Work out the finished part from the listing and answer in its coordinate system (mm). A direction names the side the tool comes from. Round coordinates to 2 decimals unless told otherwise and drop trailing zeros. Loops run counter-clockwise (first coordinate to the right, second up) from the corner with the lowest first, then second, coordinate; pieces in that order, holes last. Notation, with made-up numbers: M 9,5.25 L 44,5.25 A18 ccw 44,33.25 Z; hole C 50.25,83 d5. An arc over 180 degrees is marked long. One line per item, written item: value.
```python
from build123d import *
from build123d.topology import SkipClean

# Parameters (mm, degrees)
BOSS_EXTRUDE4_DEPTH     = 6.35
BOSS_EXTRUDE5_START     = -34.925
BOSS_EXTRUDE5_OUTLINE_R = 19.05
BOSS_EXTRUDE5_DEPTH     = 34.925
SKETCH5_R               = 6.35
CUT_EXTRUDE1_DEPTH      = 12.7
SKETCH6_R               = 6.731
CUT_EXTRUDE2_DEPTH      = 12.7
SKETCH8_W               = 34.925
SKETCH8_H               = 7.9375
BOSS_EXTRUDE6_DEPTH     = 4.7625
SKETCH9_W               = 34.925
SKETCH9_H               = 7.9375
BOSS_EXTRUDE7_DEPTH     = 4.7625
FILLET1_R               = 12.7
FILLET1_OF_MIRROR1_R    = 12.7
SKETCH10_R              = 31.75
SKETCH10_R_2            = 19.05
BOSS_EXTRUDE8_DEPTH     = 44.45
BOSS_EXTRUDE9_DEPTH     = 12.7


# Read off the part's stored shape, not the designer's step: Boss-Extrude5
with BuildPart() as part:
    # Sketch2 → Boss-Extrude4 (new body)
    with BuildSketch(Plane.XY):
        with BuildLine():
            ThreePointArc((-12.522963776, 74.083126299), (-37.56705413, 31.749689456), (0, 0))
            Line((0, 0), (0, 6.35))
            ThreePointArc((0, 6.35), (-31.75, 38.1), (0, 69.85))
            Line((0, 69.85), (0, 76.2))
            ThreePointArc((0, 76.2), (-6.350310544, 75.66705413), (-12.522963776, 74.083126299))
        make_face()
        with BuildLine():
            Line((0, 6.35), (0, 0))
            ThreePointArc((0, 0), (26.940768363, 11.159231637), (38.1, 38.1))
            ThreePointArc((38.1, 38.1), (31.054266373, 60.173571076), (12.522963776, 74.083126299))
            ThreePointArc((12.522963776, 74.083126299), (6.350310544, 75.66705413), (0, 76.2))
            Line((0, 76.2), (0, 69.85))
            ThreePointArc((0, 69.85), (22.450640303, 60.550640303), (31.75, 38.1))
            ThreePointArc((31.75, 38.1), (22.450640303, 15.649359697), (0, 6.35))
        make_face()
        with BuildLine():
            ThreePointArc((38.1, 38.1), (26.940768363, 11.159231637), (0, 0))
            Line((0, 0), (88.9, 0))
            Line((88.9, 0), (88.9, 50.8))
            Line((88.9, 50.8), (12.522963776, 74.083126299))
            ThreePointArc((12.522963776, 74.083126299), (31.054266373, 60.173571076), (38.1, 38.1))
        make_face()
        with BuildLine():
            Line((-88.9, 0), (0, 0))
            ThreePointArc((0, 0), (-37.56705413, 31.749689456), (-12.522963776, 74.083126299))
            Line((-12.522963776, 74.083126299), (-88.9, 50.8))
            Line((-88.9, 50.8), (-88.9, 0))
        make_face()
    boss_extrude4 = extrude(amount=BOSS_EXTRUDE4_DEPTH)

    # Boss-Extrude5 outline → Boss-Extrude5 (add)
    with BuildSketch(Plane(origin=(0, 0, 0), x_dir=(-1, 0, 0), z_dir=(0, 0, -1)).offset(BOSS_EXTRUDE5_START)):
        with BuildLine():
            Line((101.6, 0), (101.6, 50.8))
            Line((101.6, 50.8), (88.9, 50.8))
            Line((88.9, 50.8), (88.9, 12.7))
            Line((88.9, 12.7), (31.75, 12.7))
            Line((31.75, 12.7), (31.75, 38.1))
            ThreePointArc((31.75, 38.1), (0, 69.85), (-31.75, 38.1))
            Line((-31.75, 38.1), (-31.75, 12.7))
            Line((-31.75, 12.7), (-88.9, 12.7))
            Line((-88.9, 12.7), (-88.9, 50.8))
            Line((-88.9, 50.8), (-101.6, 50.8))
            Line((-101.6, 50.8), (-101.6, 0))
            Line((-101.6, 0), (101.6, 0))
        make_face()
        with Locations((0, 38.1)):
            Circle(BOSS_EXTRUDE5_OUTLINE_R, mode=Mode.SUBTRACT)
    boss_extrude5 = extrude(amount=BOSS_EXTRUDE5_DEPTH)

    # Sketch5 → Cut-Extrude1 (cut)
    with BuildSketch(Plane(origin=(101.6, 0, 0), x_dir=(0, 0, -1), z_dir=(1, 0, 0))):
        with Locations((-22.225, 38.1)):
            Circle(SKETCH5_R)
    cut_extrude1 = extrude(amount=-CUT_EXTRUDE1_DEPTH, mode=Mode.SUBTRACT)

    # Sketch6 → Cut-Extrude2 (cut)
    with BuildSketch(Plane.ZY.offset(101.6)):
        with Locations(Location((22.225, 38.1, 0), (0, 0, 270))):
            Circle(SKETCH6_R)
    cut_extrude2 = extrude(amount=-CUT_EXTRUDE2_DEPTH, mode=Mode.SUBTRACT)

    # Sketch8 → Boss-Extrude6 (add)
    with BuildSketch(Plane(origin=(101.6, 0, 0), x_dir=(0, 0, -1), z_dir=(1, 0, 0))):
        with Locations((-17.4625, 13.49375)):
            Rectangle(SKETCH8_W, SKETCH8_H)
    boss_extrude6 = extrude(amount=BOSS_EXTRUDE6_DEPTH)

    # Sketch9 → Boss-Extrude7 (add)
    with BuildSketch(Plane.ZY.offset(101.6)):
        with Locations((17.4625, 13.49375)):
            Rectangle(SKETCH9_W, SKETCH9_H)
    boss_extrude7 = extrude(amount=BOSS_EXTRUDE7_DEPTH)

    # Fillet1
    fillet1_edges = [part.edges().sort_by_distance(p)[0] for p in [
        (95.25, 50.8, 34.925),
        (-95.25, 50.8, 34.925),
    ]]
    fillet(fillet1_edges, radius=FILLET1_R)

    # Mirror1: Boss-Extrude4, Boss-Extrude5, Cut-Extrude1, Cut-Extrude2, Boss-Extrude6, Boss-Extrude7 across plane
    add(boss_extrude4.mirror(Plane.XY))
    add(boss_extrude5.mirror(Plane.XY))
    add(cut_extrude1.mirror(Plane.XY), mode=Mode.SUBTRACT)
    add(cut_extrude2.mirror(Plane.XY), mode=Mode.SUBTRACT)
    add(boss_extrude6.mirror(Plane.XY))
    add(boss_extrude7.mirror(Plane.XY))

    # Fillet1 of Mirror1
    fillet1_of_mirror1_edges = [part.edges().sort_by_distance(p)[0] for p in [
        (95.25, 50.8, -34.925),
        (-95.25, 50.8, -34.925),
    ]]
    fillet(fillet1_of_mirror1_edges, radius=FILLET1_OF_MIRROR1_R)

    # Sketch10 → Boss-Extrude8 (add, symmetric)
    with SkipClean():  # the faces are left unmerged after this step: merging them gives an invalid solid
        with BuildSketch(Plane.XY):
            with Locations((0, 38.1)):
                Circle(SKETCH10_R)
            with Locations((0, 38.1)):
                Circle(SKETCH10_R_2, mode=Mode.SUBTRACT)
        extrude(amount=BOSS_EXTRUDE8_DEPTH, both=True)

    # Sketch11 → Boss-Extrude9 (add)
    with SkipClean():  # the faces are left unmerged after this step: merging them gives an invalid solid
        with BuildSketch(Plane.XZ):
            Polygon((101.6, 34.925), (0, 38.1), (-101.6, 34.925), align=None)
            Polygon((-101.6, -34.925), (0, -38.1), (101.6, -34.925), align=None)
        extrude(amount=-BOSS_EXTRUDE9_DEPTH)


solid = part.part
```
1) Each of these flat-tipped pins is pushed along its axis until it touches: pin 1 (16.5 mm diameter, centred on y = 38.1, z = 22.225, fed in from +X); pin 2 (5 mm diameter, centred on y = 21, z = 29, fed in from -X); pin 3 (6 mm diameter, centred on x = 59.5, y = 30, fed in from +Z). Where does it stop, or does it pass through?
Check values:
pin 1: x = 101.6
pin 2: x = -101.6
pin 3: z = 6.35
2) Find section A-A (x = 9.5). Give the vertices of the cut face in (y, z), then the cut area to 3 significant figures.
Check values:
outline: M 0,-37.8 L 7.8,-37.8 L 7.8,-44.45 L 21.59,-44.45 L 21.59,44.45 L 7.8,44.45 L 7.8,37.8 L 0,37.8 Z; M 54.61,-44.45 L 68.4,-44.45 L 68.4,-6.35 L 75,-6.35 L 75,6.35 L 68.4,6.35 L 68.4,44.45 L 54.61,44.45 Z
area: 3,120 mm2
3) Find the intervals of material crossed by probe 1 along X at (y, z) = (18, -24); probe 2 along X at (y, z) = (15, -11); probe 3 along X at (y, z) = (27, 0), in increasing order. Write a range as from..to.
Check values:
probe 1: -101.6..-88.9, -31.75..31.75, 88.9..101.6
probe 2: -106.36..-88.9, -31.75..31.75, 88.9..106.36
probe 3: -101.6..-15.48, 15.48..101.6
4) Find section D-D (y = 64). Give the vertices of the cut face in (x, z).
Check values:
outline: M -45.6,-6.35 L -18.36,-6.35 L -18.36,-44.45 L 18.36,-44.45 L 18.36,-6.35 L 45.6,-6.35 L 45.6,6.35 L 18.36,6.35 L 18.36,44.45 L -18.36,44.45 L -18.36,6.35 L -45.6,6.35 Z
5) For faces 4 (the face through (-31.75, 25, -21)), 5 (the face through (95.339, 47.178, -31.106)), 6 (the face through (-29, 19, -34.925)), 7 (the face through (-96, 24, -34.925)), determine the directions among +Z, -Z, +X, -X, +Y, -Y from which every point of the face is accessible in a straight line to the end or side of a thin tool.
Check values:
face 4: -Z, +Y
face 5: -Z, +X, +Y
face 6: -Z, -X
face 7: -Z, -X, +Y
6) The mould has two halves that part along X. Classify faces 1 (the face through (-106.362, 14, 0)), 2 (the face through (60, 12.7, -22)), 3 (the face through (-95.161, 46.981, 31.303)): +X half, -X half, draft (parallel to the pull), parting line (faces both ways), or undercut.
Check values:
face 1: -X half
face 2: undercut
face 3: draft
